Geometry check sheet. Reference: the model listing, model coordinates, mm. A direction names the side the tool comes from. Give positions to 0.01 mm unless a question says otherwise; leave off trailing zeros. Write each loop counter-clockwise with the first axis right and the second up, starting at its lowest first coordinate (ties: lowest second). Pieces come first, ordered by that corner, then holes. Notation, with made-up numbers: (71.5, 77) - (103.5, 77) arc R15 cw to (103.5, 94) - close; hole circle Ø5 at (2, 83.5). An arc over 180 degrees is marked (long way). One line per question, with ' | ' between items. Start each with the question number.
Q1. Gauge pin test, flat ends, axial feed: P1, Ø6, axis at x = 25, z = 5.5, coming from the -Y side; P2, Ø3.5, axis at y = 20.2, z = 5, coming from the -X side; P3, Ø5, axis at x = 30.5, z = 7.5, coming from the +Y side. Record the tip position at first contact, or that the pin passes through.
Q2. Set-up check for faces 4 (the face through (24, -3, 10)), 5 (the face through (48.3, 10, 5)), 6 (the face through (44.5, -24, 5)): record each of +Z, -Z, +X, -X, +Y, -Y from which the full face is reachable in a straight line by a thin tool's end or side.
Q3. Section check A-A on y = -19. Record the boundary of the cut face in (x, z), and give its area (3 significant figures).
Q4. Release check for a two-part mould opening along Y. For faces 1 (the face through (5, 12, 5)), 2 (the face through (48.883, -8.345, 4.93)), 3 (the face through (1.335, -17.414, 5.208)) record: +Y half, -Y half, draft (parallel to the pull), parting line (faces both ways), or undercut.
Q5. Section check C-C on z = 8. Record the boundary of the cut face in (x, y), and give its area (3 significant figures).
Q6. Thickness scan on L1, parallel to Y at x = 45.55, z = 5; L2, parallel to Z at x = 48, y = -19; L3, parallel to X at y = -15, z = 3. Record the ranges inside material, lowest first. Write a range as [from, to].
Q7. Section check B-B on y = 12. Record the boundary of the cut face in (x, z).
Q8. Section check D-D on x = 37. Record the boundary of the cut face in (y, z), and give its area (3 significant figures).
Autodesk Inventor part; units mm, degrees
ref_plane "РабПлоскость1" through (24.15, 20.2, 5) normal (1, 0, 0) x (0, 0, -1)
ref_plane "YZ Plane" through (0, 0, 0) normal (1, 0, 0) x (0, 1, 0)
ref_plane "XZ Plane" through (0, 0, 0) normal (0, 1, 0) x (-1, 0, 0)
sketch "Эскиз1" plane through (0, 0, 0) normal (0, 0, 1) x (1, 0, 0)
  line L0 (0, 0) -> (5, 0)
  line L1 (5, 0) -> (5, 18)
  line L2 (5, 18) -> (0, 18)
  line L3 (0, 18) -> (0, 0)
  line L4 (0, 0) -> (24.15, 0)
  line L5 (24.15, 0) -> (24.15, -5)
  line L6 (24.15, -5) -> (0, -5)
  line L7 (0, -5) -> (0, 0)
  dimension "d0" = 5
  dimension "d1" = 18
  dimension "d2" = 24.15
  dimension "d3" = 5
extrude "Выдавливание1" add sketch "Эскиз1" along normal blind 10
sketch "Эскиз4" plane through (0, 18, 0) normal (0, 1, 0) x (1, 0, 0)
  line L0 (0, 0) -> (0, -10)
  line L1 (0, 0) -> (0, -10)
  line L2 (5, 0) -> (0, 0)
  line L3 (0, 0) -> (0, -10)
  line L4 (5, -10) -> (0, -10)
  line L5 (5, 0) -> (5, -10)
extrude "Выдавливание2" add sketch "Эскиз4" along normal blind 7.2
fillet "Сопряжение1" radius 5 2 edges at (2.5, 25.2, 10) (2.5, 25.2, 0)
sketch "Эскиз5" plane through (5, 0, 10) normal (1, 0, 0) x (0, 0, -1)
  line L0 (0, -5) -> (0, -5)
  line L1 (10, -5) -> (10, -5)
  arc A0 (10, 20.2) -> (0, 20.2) centre (5, 20.2) ccw
  point P0 (10, 0)
hole "Отверстие2" at (5, 20.2, 5) direction (-1, 0, 0) diameter 3.2 depth 5
mirror "Зеркальное отражение1" about plane through (24.15, -5, 0) normal (1, 0, 0)
sketch "Эскиз9" plane through (0, 0, 0) normal (0, 0, -1) x (-1, 0, 0)
  line L0 (-48.3, 20.2) -> (-48.3, -5)
  line L1 (-48.3, -5) -> (-43.3, -5)
  line L2 (-43.3, -5) -> (-43.3, -4.289)
  line L3 (-43.3, -4.289) -> (-48.3, -4.289)
  line L4 (-48.3, -4.289) -> (-48.3, -5)
  line L5 (-48.3, -4.289) -> (-43.3508, -5)
  line L6 (-43.3508, -5) -> (-44.5, -13)
  line L7 (-44.5, -13) -> (-49.4492, -12.289)
  line L8 (-49.4492, -12.289) -> (-48.3, -4.289)
  line L9 (-44.5, -13) -> (-49.5, -13)
  line L10 (-49.5, -13) -> (-49.5, -34)
  line L11 (-49.5, -34) -> (-44.5, -34)
  line L12 (-44.5, -34) -> (-44.5, -13)
  line L13 (0, -5) -> (-48.3, -5)
  line L14 (-49.4492, -12.289) -> (-49.5, -13)
  point P0 (0, 0)
  point P1 (-43.3, -5.581)
  point P2 (-46.5, -13.5979)
  dimension "d39" = 5
  dimension "d45" = 5
  dimension "d47" = 5
  dimension "d66" = 29
  dimension "d68" = 21
  dimension "d71" = 1.2
extrude "Выдавливание4" add sketch "Эскиз9" against normal blind 10
sketch "Эскиз10" plane through (49.5, -34, 0) normal (1, 0, 0) x (0, 0, -1)
  line L0 (0, 0) -> (-10, 0)
  line L1 (-5, 0) -> (-5, 5)
  line L2 (-5, 5) -> (-5, 15)
  point P0 (0, 34)
  dimension "d48" = 5
  dimension "d49" = 10
hole "Отверстие5" at (49.5, -19, 5) at (49.5, -29, 5) direction (-1, 0, 0) diameter 3.2 end through all
ref_plane "РабПлоскость1" through (24.15, 20.2, 5) normal (1, 0, 0) x (0, 0, -1)
mirror "Зеркальное отражение2" about plane through (24.15, 20.2, 5) normal (1, 0, 0) of "Выдавливание4", "Отверстие5"
equation "\"d63\" = Толщина"
equation "\"Радиус_гибки\" = Толщина"
equation "\"Ширина_просечки\" = Толщина"
equation "\"Глубина_просечки\" = 0.5 * Толщина"
equation "\"Размер_просечки\" = 4 * Толщина"
equation "\"Мин_остаток\" = 2 * Толщина"
equation "\"Радиус_перехода\" = Радиус_гибки"
equation "\"Радиус_Якоби\" = Толщина"
equation "\"Размер_зазора\" = Толщина"
properties part number "Стойка для камеры"
Working result:
1) P1: stops at y = -5 | P2: stops at x = 0 | P3: stops at y = 0
2) face 4: +Z, +X, -X, +Y, -Y | face 5: +Z, -Z, +X, +Y | face 6: +Z, -Z, -Y
3) outline: (-1.2, 0) - (3.8, 0) - (3.8, 3.4) - (-1.2, 3.4) - close; (-1.2, 6.6) - (3.8, 6.6) - (3.8, 10) - (-1.2, 10) - close; (44.5, 0) - (49.5, 0) - (49.5, 3.4) - (44.5, 3.4) - close; (44.5, 6.6) - (49.5, 6.6) - (49.5, 10) - (44.5, 10) - close | area: 68.0 mm2
4) face 1: draft | face 2: +Y half | face 3: undercut
5) outline: (-1.2, -34) - (3.8, -34) - (3.8, -13) - (4.95, -5) - (43.35, -5) - (44.5, -13) - (44.5, -34) - (49.5, -34) - (49.5, -13) - (49.45, -12.29) - (48.3, -4.29) - (48.3, 24.2) - (43.3, 24.2) - (43.3, 0) - (5, 0) - (5, 24.2) - (0, 24.2) - (0, -4.29) - (-1.15, -12.29) - (-1.2, -13) - close | area: 774 mm2
6) L1: y = [-34, -30.6], [-27.4, -20.6], [-17.4, 18.6], [21.8, 25.2] | L2: z = [0, 3.4], [6.6, 10] | L3: x = [-1.2, 3.8], [44.5, 49.5]
7) outline: (0, 0) - (5, 0) - (5, 10) - (0, 10) - close; (43.3, 0) - (48.3, 0) - (48.3, 10) - (43.3, 10) - close
8) outline: (-5, 0) - (0, 0) - (0, 10) - (-5, 10) - close | area: 50.0 mm2
